Check sheet for the drawn part. Datum: minimum x, y, z corner. Units: mm. A direction names the side the tool comes from. Coordinates: 2 decimals unless noted, no trailing zeros. Order: outer loops, then holes, each group sorted by start corner. A loop starts at its lowest first (then second) coordinate and runs counter-clockwise, first axis right, second up. Notation, with made-up numbers: M 43,-24.5 L 75,-24.5 A17 ccw 75,2.5 Z; hole C -25,0 d3. An arc over 180 degrees is marked long. Answer in a Markdown table with one row per item. Add a question column.
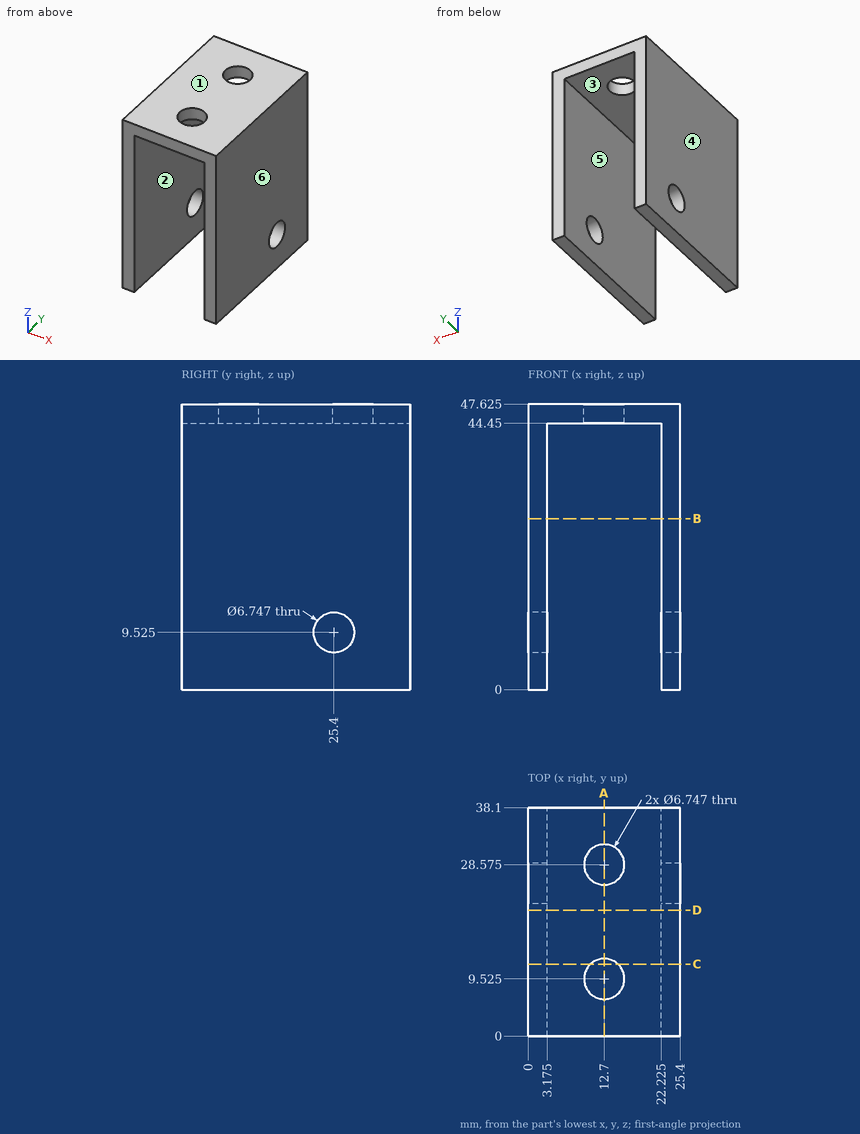
1. Set-up check for the marked faces 5 and 6: record each of +Z, -Z, +X, -X, +Y, -Y from which the full face is reachable in a straight line by a thin tool's end or side.
2. Go/stop test with a flat-tipped pin: pin 1 Ø9.5 at (x, y) = (10.5, 22) entering from -Z. Record where the tip stops, or that it passes through.
3. Section check A-A on x = 12.7. State how many separate pieces and enclosed holes the cut face has, then the cut area to 3 significant figures.
4. Section check C-C on y = 12. Enter the section's corners in (x, z) (3 decimals), then the cut area to 3 significant figures.
5. Release check for a two-part mould opening along X. For the marked faces 1, 2, 3 and 4 record: released by +X, released by -X, zero draft, split by the parting line, or undercut.
6. Scan lines: line 1 (Y direction, x = 12.7, z = 46.7); line 2 (X direction, y = 30.5, z = 16) (3 decimals); line 3 (Z direction, x = 2.2, y = 25.4) (1 decimal). Record each from-to range of solid material in increasing order.
7. Section check D-D on y = 21. Enter the section's corners in (x, z) (3 decimals), then the cut area to 3 significant figures.
8. Section check B-B on z = 28.5. Enter the section's corners in (x, y) (3 decimals), then the cut area to 3 significant figures.
Result sheet:
| question | item | result |
|---|---|---|
| 1 | face 5 | -Z, +Y, -Y |
| 1 | face 6 | +Z, -Z, +X, +Y, -Y |
| 2 | pin 1 | z = 44.45 |
| 3 | separate pieces | 3 |
| 3 | enclosed holes | 0 |
| 3 | area | 78.1 mm^2 |
| 4 | outline | M 0,0 L 3.175,0 L 3.175,44.45 L 10.408,44.45 L 10.408,47.625 L 0,47.625 Z; M 14.992,44.45 L 22.225,44.45 L 22.225,0 L 25.4,0 L 25.4,47.625 L 14.992,47.625 Z |
| 4 | area | 348 mm^2 |
| 5 | face 1 | zero draft |
| 5 | face 2 | undercut |
| 5 | face 3 | undercut |
| 5 | face 4 | released by -X |
| 6 | line 1 | 0 to 6.15, 12.9 to 25.2, 31.95 to 38.1 |
| 6 | line 2 | 0 to 3.175, 22.225 to 25.4 |
| 6 | line 3 | 0 to 6.2, 12.9 to 47.6 |
| 7 | outline | M 0,0 L 3.175,0 L 3.175,44.45 L 22.225,44.45 L 22.225,0 L 25.4,0 L 25.4,47.625 L 0,47.625 Z |
| 7 | area | 363 mm^2 |
| 8 | outline | M 0,0 L 3.175,0 L 3.175,38.1 L 0,38.1 Z; M 22.225,0 L 25.4,0 L 25.4,38.1 L 22.225,38.1 Z |
| 8 | area | 242 mm^2 |
